Read the model definition and answer for the solid it produces. Units are mm, in the model's axes. A direction names the side the tool comes from. Coordinates: 2 decimals unless noted, no trailing zeros. Loops run counter-clockwise (first coordinate to the right, second up) from the corner with the lowest first, then second, coordinate; pieces in that order, holes last. Notation, with made-up numbers: (-17, 34) - (-4, 34) arc R8 cw to (-4, 42) - close; hole circle Ø3 at (15.5, -10.75). An arc over 180 degrees is marked (long way). Use one line per item in the form item = value.
Autodesk Inventor part; units mm, degrees
ref_plane "Płaszczyzna konstrukcyjna1" through (0, 0, 8) normal (0, 0, 1) x (1, 0, 0)
ref_plane "YZ Plane" through (0, 0, 0) normal (1, 0, 0) x (0, 1, 0)
ref_plane "XZ Plane" through (0, 0, 0) normal (0, 1, 0) x (-1, 0, 0)
sketch "Szkic1" plane through (0, 0, 0) normal (0, 0, 1) x (1, 0, 0)
  line L0 (0, 0) -> (33.5, 0)
  line L1 (0, 0) -> (-33.5, 0)
  circle A0 centre (0, 18) radius 5
  line L2 (-33.5, 0) -> (-33.5, 6)
  line L3 (33.5, 6) -> (33.5, 0)
  line L4 (-19.5, 6) -> (-26.5, 6)
  line L5 (19.5, 6) -> (26.5, 6)
  line L6 (-26.5, 6) -> (-19.5, 6)
  line L7 (26.5, 6) -> (19.5, 6)
  line L8 (0, 18) -> (-14.722432, 26.5) construction
  line L9 (0, 18) -> (0, 35) construction
  line L10 (0, 18) -> (14.722432, 26.5) construction
  line L11 (0, 18) -> (0, 35) construction
  arc A1 (19.5, 6) -> (14.722432, 26.5) centre (-44.369926, 1.921691) ccw
  line L12 (-33.5, 6) -> (-19.5, 6)
  line L13 (19.5, 6) -> (33.5, 6)
  arc A2 (-14.722432, 26.5) -> (-19.5, 6) centre (44.369926, 1.921691) ccw
  line L14 (-19.5, 6) -> (19.5, 6)
  line L15 (-14.722432, 26.5) -> (-14.722432, 6)
  line L16 (14.722432, 26.5) -> (14.722432, 6)
  arc A3 (0, 35) -> (-14.722432, 26.5) centre (0, 18) ccw
  arc A4 (14.722432, 26.5) -> (0, 35) centre (0, 18) ccw
  dimension "d0" = 33.5
  dimension "d1" = 33.5
  dimension "d2" = 35
  dimension "d4" = 10
  dimension "d5" = 6
  dimension "d9" = 7
  dimension "d10" = 7
  dimension "d11" = 60
  dimension "d12" = 60
  dimension "d14" = 64
  dimension "d15" = 64
sketch "Szkic1 outline for Wyciągnięcie proste1" plane through (0, 0, 0) normal (0, 0, 1) x (1, 0, 0)
  arc A0 (19.5, 6) -> (14.722432, 26.5) centre (-44.369926, 1.921691) ccw
  arc A1 (14.722432, 26.5) -> (-14.722432, 26.5) centre (0, 18) ccw
  arc A2 (-14.722432, 26.5) -> (-19.5, 6) centre (44.369926, 1.921691) ccw
  line L0 (-19.5, 6) -> (-33.5, 6)
  line L1 (-33.5, 6) -> (-33.5, 0)
  line L2 (-33.5, 0) -> (33.5, 0)
  line L3 (33.5, 0) -> (33.5, 6)
  line L4 (33.5, 6) -> (19.5, 6)
  circle A3 centre (0, 18) radius 5
extrude "Wyciągnięcie proste1" add sketch "Szkic1 outline for Wyciągnięcie proste1" along normal blind 16
sketch "Szkic2" plane through (-33.5, 0, 0) normal (0, -1, 0) x (1, 0, 0)
  circle A0 centre (7, 8) radius 3
  circle A1 centre (60, 8) radius 3
sketch "Szkic2 outline for Wyciągnięcie proste2" plane through (-33.5, 0, 0) normal (0, -1, 0) x (1, 0, 0)
  circle A0 centre (7, 8) radius 3
  circle A1 centre (60, 8) radius 3
extrude "Wyciągnięcie proste2" cut sketch "Szkic2 outline for Wyciągnięcie proste2" against normal up to next
ref_plane "Płaszczyzna konstrukcyjna1" through (0, 0, 8) normal (0, 0, 1) x (1, 0, 0)
sketch "Szkic3" plane through (0, 0, 8) normal (0, 0, 1) x (1, 0, 0)
  circle A0 centre (0, 18) radius 5
  circle A1 centre (0, 18) radius 8
  point P0 (0, 0)
  dimension "d28" = 16
sketch "Szkic3 outline for Wyciągnięcie proste3" plane through (0, 0, 8) normal (0, 0, 1) x (1, 0, 0)
  circle A0 centre (0, 18) radius 8
  circle A1 centre (0, 18) radius 5
extrude "Wyciągnięcie proste3" add sketch "Szkic3 outline for Wyciągnięcie proste3" along normal blind 10
sketch "Szkic4" plane through (0, 0, 16) normal (0, 0, 1) x (1, 0, 0)
  arc A0 (-14.722432, 26.5) -> (-19.5, 6) centre (44.369926, 1.921691) ccw
  arc A1 (14.722432, 26.5) -> (-14.722432, 26.5) centre (0, 18) ccw
  arc A2 (19.5, 6) -> (14.722432, 26.5) centre (-44.369926, 1.921691) ccw
  arc A3 (-16.750014, 20.904656) -> (16.750014, 20.904656) centre (0, 18) ccw
  circle A4 centre (0, 18) radius 14.5
  circle A5 centre (0, 18) radius 8
  point P0 (0, 0)
  dimension "d31" = 29
sketch "Szkic4 outline for Wyciągnięcie proste4" plane through (0, 0, 16) normal (0, 0, 1) x (1, 0, 0)
  circle A0 centre (0, 18) radius 14.5
  circle A1 centre (0, 18) radius 8
extrude "Wyciągnięcie proste4" cut sketch "Szkic4 outline for Wyciągnięcie proste4" against normal blind 5
sketch "Szkic5" plane through (0, 0, 0) normal (0, 0, -1) x (-1, 0, 0)
  circle A0 centre (0, 18) radius 5
  circle A1 centre (0, 18) radius 8
  arc A2 (14.722432, 26.5) -> (-14.722432, 26.5) centre (0, 18) ccw
  arc A3 (19.5, 6) -> (14.722432, 26.5) centre (-44.369926, 1.921691) ccw
  arc A4 (-14.722432, 26.5) -> (-19.5, 6) centre (44.369926, 1.921691) ccw
  arc A5 (-14.722432, 26.5) -> (-19.5, 6) centre (44.369926, 1.921691) ccw
  arc A6 (19.5, 6) -> (14.722432, 26.5) centre (-44.369926, 1.921691) ccw
  arc A7 (-16.750014, 20.904656) -> (16.750014, 20.904656) centre (0, 18) ccw
  circle A8 centre (0, 18) radius 14.5
  point P0 (0, 0)
  dimension "d34" = 16
  dimension "d35" = 29
sketch "Szkic5 outline for Wyciągnięcie proste5" plane through (0, 0, 0) normal (0, 0, -1) x (-1, 0, 0)
  circle A0 centre (0, 18) radius 14.5
  circle A1 centre (0, 18) radius 8
extrude "Wyciągnięcie proste5" cut sketch "Szkic5 outline for Wyciągnięcie proste5" against normal blind 5
sketch "Szkic6" plane through (0, 18, 0) normal (0, 0, -1) x (-1, 0, 0)
  circle A0 centre (0, 0) radius 8
  circle A1 centre (0, 0) radius 5
  point P0 (0, -18)
sketch "Szkic6 outline for Wyciągnięcie proste6" plane through (0, 18, 0) normal (0, 0, -1) x (-1, 0, 0)
  circle A0 centre (0, 0) radius 8
  circle A1 centre (0, 0) radius 5
extrude "Wyciągnięcie proste6" cut sketch "Szkic6 outline for Wyciągnięcie proste6" against normal blind 4
fillet "Zaokrąglenie1" radius 5 4 edges at (-33.5, 3, 16) (-33.5, 3, 0) (33.5, 3, 16) (33.5, 3, 0)
fillet "Zaokrąglenie2" radius 2 14 edges at (17.9598, 16.4478, 16) (0, 35, 16) (-17.9598, 16.4478, 16) (32.0355, 6, 14.5355) (33.5, 6, 8) (32.0355, 6, 1.4645) (-24, 6, 0) (24, 6, 16) (-32.0355, 6, 14.5355) (-33.5, 6, 8) (-32.0355, 6, 1.4645) (0, 35, 0) (-17.9598, 16.4478, 0) (17.9598, 16.4478, 0)
properties part number "Łożysko w obudowie aluminiowej 10mm KP000"
Item 1: The part is cut by section C-C on x = 26.5. Give the vertices of the cut face in (y, z).
Results below:
outline = (0, 0) - (4, 0) arc R2 ccw to (6, 2) - (6, 5) - (0, 5) - close; (0, 11) - (6, 11) - (6, 14) arc R2 ccw to (4, 16) - (0, 16) - close
Item 2: Each of these flat-tipped pins is pushed along its axis until it touches: P1, Ø3, axis at y = 18, z = 2, coming from the +X side; P2, Ø3.5, axis at x = -27, z = 10, coming from the +Y side; P3, Ø3, axis at y = 18, z = 5.5, coming from the -X side. Where does it stop, or does it pass through?
Results below:
P1 = 17.95
P2 = 6
P3 = -17.95
Item 3: Which of the six approach directions +Z, -Z, +X, -X, +Y, -Y give full straight-line access (tool end or side, diameter ignored) to faces 4 (the cylindrical face through (7.795, 30.226, 13.535)), 5 (the flat face through (-23, 6, 8)), 6 (the cylindrical face through (1.73, 10.19, 4.49)), 7 (the cylindrical face through (32, 2.03, 14.57)), 8 (the cylindrical face through (23.12, 5.4, 0.57))?
Results below:
face_4 = +Z
face_5 = +Z, -Z, -X, +Y
face_6 = -Z
face_7 = +Z, +X, +Y, -Y
face_8 = -Z, +X, +Y
Item 4: The part is cut by section D-D on z = 13.25. Count the separate pieces of the cut face and the enclosed holes in it, plus the area to 3 significant figures.
Results below:
separate_pieces = 2
enclosed_holes = 2
area = 759 mm²
Item 5: The part is cut by section A-A on x = 0. Give the vertices of the cut face in (y, z), plus the area to 3 significant figures.
Results below:
outline = (0, 0) - (3.5, 0) - (3.5, 5) - (10, 5) - (10, 4) - (13, 4) - (13, 18) - (10, 18) - (10, 11) - (3.5, 11) - (3.5, 16) - (0, 16) - close; (23, 4) - (26, 4) - (26, 5) - (32.5, 5) - (32.5, 0) - (33, 0) arc R2 ccw to (35, 2) - (35, 14) arc R2 ccw to (33, 16) - (32.5, 16) - (32.5, 11) - (26, 11) - (26, 18) - (23, 18) - close
area = 256 mm²
Item 6: The part is cut by section B-B on z = 6. Give the vertices of the cut face in (x, y).
Results below:
outline = (-33.5, 0) - (-28.74, 0) - (-28.74, 6) - (-31.5, 6) arc R2 ccw to (-33.5, 4) - close; (-24.26, 0) - (24.26, 0) - (24.26, 6) - (19.5, 6) arc R64 ccw to (14.72, 26.5) arc R17 ccw to (-14.72, 26.5) arc R64 ccw to (-19.5, 6) - (-24.26, 6) - close; (28.74, 0) - (33.5, 0) - (33.5, 4) arc R2 ccw to (31.5, 6) - (28.74, 6) - close; hole circle Ø10 at (0, 18)
Item 7: Find the intervals of material crossed by L1, parallel to Y at x = -3, z = 14.75; L2, parallel to Y at x = 3.5, z = 15.75; L3, parallel to Z at x = 16, y = 11.5, in increasing order.
Results below:
L1 = 0 to 3.81, 10.58 to 14, 22 to 25.42, 32.19 to 34.58
L2 = 0 to 3.93, 10.81 to 14.43, 21.57 to 25.19, 32.07 to 33.58
L3 = 0 to 16
Item 8: For a pull along Y with two mould halves and no side action, classify faces 1 (the cylindrical face through (-17.993, 16.304, 7.916)), 2 (the flat face through (-6, 12, 5)), 3 (the cylindrical face through (-32.07, 1.97, 1.5)) as +Y half, -Y half, draft (parallel to the pull), parting line (faces both ways), or undercut.
Results below:
face_1 = +Y half
face_2 = undercut
face_3 = draft
